```python
from build123d import *

# Parameters (mm, degrees)
SKETCH1_R           = 36
SKETCH1_R_2         = 30.6
BOSS_EXTRUDE1_DEPTH = 5
SKETCH2_R           = 32.6
CUT_EXTRUDE1_DEPTH  = 3.5


with BuildPart() as part:
    # Sketch1 → Boss-Extrude1 (new body, symmetric)
    with BuildSketch(Plane(origin=(0, 0, 0), x_dir=(1, 0, 0), z_dir=(0, 1, 0))):
        Circle(SKETCH1_R)
        Circle(SKETCH1_R_2, mode=Mode.SUBTRACT)
    extrude(amount=BOSS_EXTRUDE1_DEPTH, both=True)

    # Sketch2 → Cut-Extrude1 (cut, symmetric)
    with BuildSketch(Plane(origin=(0, 0, 0), x_dir=(1, 0, 0), z_dir=(0, 1, 0))):
        Circle(SKETCH2_R)
    extrude(amount=CUT_EXTRUDE1_DEPTH, both=True, mode=Mode.SUBTRACT)


solid = part.part
```
For this review, take the finished solid that the model builds, in its own axes (mm). A direction names the side the tool comes from. Round coordinates to 2 decimals unless told otherwise and drop trailing zeros. Write each loop counter-clockwise with the first axis right and the second up, starting at its lowest first coordinate (ties: lowest second). Pieces come first, ordered by that corner, then holes. Notation, with made-up numbers: (64, 20) -> (85, 20) arc R23 ccw to (85, 48) -> close; hole circle Ø10 at (30, 78). An arc over 180 degrees is marked (long way). One line per question, with ' | ' between items. Start each with the question number.
1) Add section A-A (x = 0). Write out the cut boundary in (y, z).
2) For pin 1 Ø2 at (y, z) = (1, 8.5) entering from -X; pin 2 Ø6 at (y, z) = (1.5, 4) entering from +X; pin 3 Ø5 at (x, y) = (27, 0.5) entering from +Z, all flat-tipped, find the tip position at first contact; note any pin that passes through.
3) Machinability: for faces 1 (the cylindrical face through (-25.9, 0, 19.8)), 2 (the flat face through (-16.2, 5, 26.5)), which of the approach directions +Z, -Z, +X, -X, +Y, -Y give a long, thin tool a straight path to every point of the face, cutting with its end or side? Answer none if there is none.
4) Add section C-C (y = 0). Write out the cut boundary in (x, z).
5) Add section B-B (z = 0). Write out the cut boundary in (x, y), and give its area (3 significant figures).
6) Wall thickness on line 1 along Z through (x, y) = (0, -4.6); line 2 along Z through (x, y) = (0, 0.5): over which ranges is each line inside the solid? List them lowest first.
7) Mouldability with a two-part tool opening along Z and no side actions: class faces 3 (the cylindrical face through (-4.686, 0.07, -35.694)), 4 (the flat face through (-16.2, -5, 26.5)), 5 (the cylindrical face through (-6.633, 4.24, 29.872)) as +Z half, -Z half, draft (parallel to the pull), parting line (faces both ways), or undercut.
Reported:
1) outline: (-5, -36) -> (5, -36) -> (5, -30.6) -> (3.5, -30.6) -> (3.5, -32.6) -> (-3.5, -32.6) -> (-3.5, -30.6) -> (-5, -30.6) -> close; (-5, 30.6) -> (-3.5, 30.6) -> (-3.5, 32.6) -> (3.5, 32.6) -> (3.5, 30.6) -> (5, 30.6) -> (5, 36) -> (-5, 36) -> close
2) pin 1: stops at x = -35.21 | pin 2: stops at x = 35.99 | pin 3: stops at z = 26.38
3) face 1: none | face 2: +Z, -Z, +X, -X, +Y
4) outline: circle Ø72 at (0, 0); hole circle Ø65.2 at (0, 0)
5) outline: (-36, -5) -> (-30.6, -5) -> (-30.6, -3.5) -> (-32.6, -3.5) -> (-32.6, 3.5) -> (-30.6, 3.5) -> (-30.6, 5) -> (-36, 5) -> close; (30.6, -5) -> (36, -5) -> (36, 5) -> (30.6, 5) -> (30.6, 3.5) -> (32.6, 3.5) -> (32.6, -3.5) -> (30.6, -3.5) -> close | area: 80.0 mm²
6) line 1: z = -36 to -30.6, 30.6 to 36 | line 2: z = -36 to -32.6, 32.6 to 36
7) face 3: parting line | face 4: draft | face 5: undercut
